```python
from build123d import *

# Parameters (mm, degrees)
SKETCH_1_R                  = 18
SKETCH_1_R_2                = 1.7
F_04_BEARING_RETAINER_DEPTH = 2.8


with BuildPart() as part:
    # Эскиз1 → 04_Bearing_retainer (new body)
    with BuildSketch(Plane.XY):
        Polygon((-21, -36), (21, -36), (36, -21), (36, 21), (21, 36), (-21, 36), (-36, 21), (-36, -21), align=None)
        Circle(SKETCH_1_R, mode=Mode.SUBTRACT)
        with Locations((0, 29)):
            Circle(SKETCH_1_R_2, mode=Mode.SUBTRACT)
        with Locations((0, -29)):
            Circle(SKETCH_1_R_2, mode=Mode.SUBTRACT)
        with Locations((-29, 0)):
            Circle(SKETCH_1_R_2, mode=Mode.SUBTRACT)
    extrude(amount=F_04_BEARING_RETAINER_DEPTH)


solid = part.part
```
Source: CAD feature listing. Evaluate the final solid. Frame: model axes, mm. Round coordinates to 2 decimals unless told otherwise and drop trailing zeros. Order: outer loops, then holes, each group sorted by start corner. A loop starts at its lowest first (then second) coordinate and runs counter-clockwise, first axis right, second up. Notation, with made-up numbers: (-19, 19.5) -> (35, 19.5) arc R29 cw to (35, 50.5) -> close; hole circle Ø10 at (88.25, 19.5). An arc over 180 degrees is marked (long way). One line per item, written item: value. Start each with the question number.
Q1. Section query C-C (x = 0). Return the cut outline in (y, z), plus the area to 3 significant figures.
Q2. Material intervals for probe 1 along Y at (x, z) = (0, 0.7); probe 2 along X at (y, z) = (-12.5, 0.15); probe 3 along X at (y, z) = (-10.5, 1.25), sorted ascending.
Q3. Section query B-B (y = 0). Return the cut outline in (x, z).
Q4. Section query D-D (z = 1.8). Return the cut outline in (x, y), plus the area to 3 significant figures.
Q5. Draft query along Y for faces 1 (the flat face through (28, -29, 1)), 2 (the cylindrical face through (-27.43, -0.65, 1.38)), 3 (the flat face through (-17, -7, 2.8)). Return one class per face: pulls with the +Y half, pulls with the -Y half, needs draft (parallel to the pull), parting line crosses it, or undercut.
Q6. Section query A-A (y = 29). Return the cut outline in (x, z), plus the area to 3 significant figures.
Findings below:
1. outline: (-36, 0) -> (-30.7, 0) -> (-30.7, 2.8) -> (-36, 2.8) -> close; (-27.3, 0) -> (-18, 0) -> (-18, 2.8) -> (-27.3, 2.8) -> close; (18, 0) -> (27.3, 0) -> (27.3, 2.8) -> (18, 2.8) -> close; (30.7, 0) -> (36, 0) -> (36, 2.8) -> (30.7, 2.8) -> close
1. area: 81.8 mm²
2. probe 1: -36 to -30.7, -27.3 to -18, 18 to 27.3, 30.7 to 36
2. probe 2: -36 to -12.95, 12.95 to 36
2. probe 3: -36 to -14.62, 14.62 to 36
3. outline: (-36, 0) -> (-30.7, 0) -> (-30.7, 2.8) -> (-36, 2.8) -> close; (-27.3, 0) -> (-18, 0) -> (-18, 2.8) -> (-27.3, 2.8) -> close; (18, 0) -> (36, 0) -> (36, 2.8) -> (18, 2.8) -> close
4. outline: (-36, -21) -> (-21, -36) -> (21, -36) -> (36, -21) -> (36, 21) -> (21, 36) -> (-21, 36) -> (-36, 21) -> close; hole circle Ø3.4 at (-29, 0); hole circle Ø36 at (0, 0); hole circle Ø3.4 at (0, -29); hole circle Ø3.4 at (0, 29)
4. area: 3,690 mm²
5. face 1: pulls with the -Y half
5. face 2: undercut
5. face 3: needs draft
6. outline: (-28, 0) -> (-1.7, 0) -> (-1.7, 2.8) -> (-28, 2.8) -> close; (1.7, 0) -> (28, 0) -> (28, 2.8) -> (1.7, 2.8) -> close
6. area: 147 mm²
